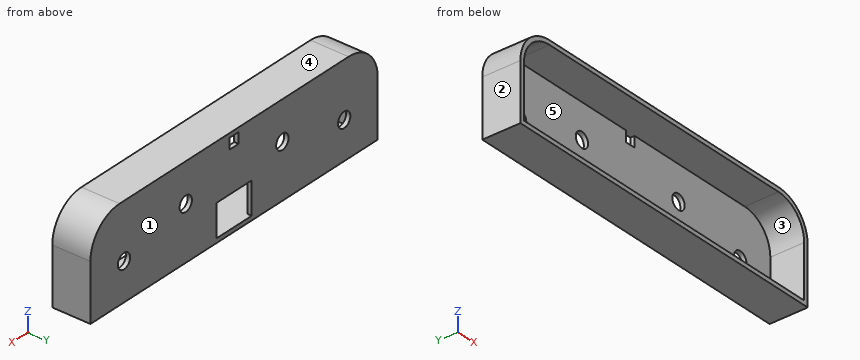
```python
from build123d import *

# Parameters (mm, degrees)
SKETCH1_W           = 162.7
SKETCH1_H           = 43
BOSS_EXTRUDE2_DEPTH = 17.75
FILLET2_R           = 16.5
SHELL1_T            = -2
SKETCH2_R           = 3.5
CUT_EXTRUDE1_DEPTH  = 86.994970783
SKETCH5_W           = 20
SKETCH5_H           = 15
CUT_EXTRUDE2_DEPTH  = 86.994970783
SKETCH6_W           = 5
SKETCH6_H           = 5
CUT_EXTRUDE3_DEPTH  = 86.994970783


with BuildPart() as part:
    # Sketch1 → Boss-Extrude2 (new body)
    with BuildSketch(Plane(origin=(0, 0, 0), x_dir=(1, 0, 0), z_dir=(0, 1, 0))):
        Rectangle(SKETCH1_W, SKETCH1_H)
    extrude(amount=BOSS_EXTRUDE2_DEPTH)

    # Fillet2
    fillet2_edges = [part.edges().sort_by_distance(p)[0] for p in [
        (81.35, 8.875, 21.5),
        (-81.35, 8.875, 21.5),
    ]]
    fillet(fillet2_edges, radius=FILLET2_R)

    # Shell1
    shell1_openings = [part.faces().sort_by_distance(p)[0] for p in [
        (0, 0, -0.302595299),
    ]]
    offset(amount=SHELL1_T, openings=shell1_openings, kind=Kind.INTERSECTION)

    # Sketch2 → Cut-Extrude1 (cut, through all)
    with BuildSketch(Plane(origin=(0, 17.75, 0), x_dir=(1, 0, 0), z_dir=(0, 1, 0))):
        with Locations(Location((-62.35, 4, 0), (0, 0, 270))):
            Circle(SKETCH2_R)
        with Locations(Location((-27.35, -3.5, 0), (0, 0, 270))):
            Circle(SKETCH2_R)
        with Locations(Location((27.35, -3.5, 0), (0, 0, 90))):
            Circle(SKETCH2_R)
        with Locations(Location((62.35, 4, 0), (0, 0, 90))):
            Circle(SKETCH2_R)
    extrude(amount=-CUT_EXTRUDE1_DEPTH, mode=Mode.SUBTRACT)

    # Sketch5 → Cut-Extrude2 (cut, through all)
    with BuildSketch(Plane(origin=(0, 17.75, 0), x_dir=(1, 0, 0), z_dir=(0, 1, 0))):
        with Locations((0, 12)):
            Rectangle(SKETCH5_W, SKETCH5_H)
    extrude(amount=-CUT_EXTRUDE2_DEPTH, mode=Mode.SUBTRACT)

    # Sketch6 → Cut-Extrude3 (cut, through all)
    with BuildSketch(Plane(origin=(0, 17.75, 0), x_dir=(1, 0, 0), z_dir=(0, 1, 0))):
        with Locations((0, -17)):
            Rectangle(SKETCH6_W, SKETCH6_H)
    extrude(amount=-CUT_EXTRUDE3_DEPTH, mode=Mode.SUBTRACT)


solid = part.part
```
Input: part model. Units: mm. Frame: model coordinates. Face numbers are marked on the shaded views. A direction names the side the tool comes from. Coordinates: 2 decimals unless noted, no trailing zeros. Write each loop counter-clockwise with the first axis right and the second up, starting at its lowest first coordinate (ties: lowest second). Pieces come first, ordered by that corner, then holes.
1) Section A-A on z = 3.5. Output: boundary loops of the cut face in (x, y).
2) Section B-B on x = -62.35. Output: boundary loops of the cut face in (y, z), and give its area (3 significant figures).
3) Section C-C on z = -12. Output: boundary loops of the cut face in (x, y), and give its area (3 significant figures).
4) Set-up query: the marked faces 4 and 5. Return all of +Z, -Z, +X, -X, +Y, -Y with unobstructed straight access to the full face (end or side cutting, diameter ignored); none if empty.
5) Section D-D on y = 3. Output: boundary loops of the cut face in (x, z).
6) Pin query (flat end, axial travel): pin 1 Ø1 at (y, z) = (16.5, 16.5) entering from -X; pin 2 Ø11.5 at (x, z) = (-39.5, 9.5) entering from -Y; pin 3 Ø4 at (x, z) = (-62.35, -4) entering from -Y. Return the tip coordinate at first contact, or that it passes through.
7) Mould query, pull axis X, two halves, no side actions, for the marked faces 1, 2 and 3. Classes: pulls with the +X half, pulls with the -X half, needs draft (parallel to the pull), parting line crosses it, or undercut.
8) Material intervals for line 1 along X through (y, z) = (16.8, -4); line 2 along X through (y, z) = (16.3, 3.5); line 3 along Z through (x, y) = (38, 13.75), sorted ascending.
Check result:
1. outline: (-81.35, 0) - (-79.35, 0) - (-79.35, 15.75) - (-30.85, 15.75) - (-30.85, 17.75) - (-81.35, 17.75) - close; (-23.85, 15.75) - (23.85, 15.75) - (23.85, 17.75) - (-23.85, 17.75) - close; (30.85, 15.75) - (79.35, 15.75) - (79.35, 0) - (81.35, 0) - (81.35, 17.75) - (30.85, 17.75) - close
2. outline: (0, -21.5) - (17.75, -21.5) - (17.75, -7.5) - (15.75, -7.5) - (15.75, -19.5) - (0, -19.5) - close; (0, 19.5) - (15.75, 19.5) - (15.75, -0.5) - (17.75, -0.5) - (17.75, 21.5) - (0, 21.5) - close
2. area: 135 mm2
3. outline: (-81.35, 0) - (-79.35, 0) - (-79.35, 15.75) - (-10, 15.75) - (-10, 17.75) - (-81.35, 17.75) - close; (10, 15.75) - (79.35, 15.75) - (79.35, 0) - (81.35, 0) - (81.35, 17.75) - (10, 17.75) - close
3. area: 348 mm2
4. face 4: +Z, +X, -X, +Y, -Y
4. face 5: -Y
5. outline: (-81.35, -21.5) - (81.35, -21.5) - (81.35, 5) arc R16.5 ccw to (64.85, 21.5) - (-64.85, 21.5) arc R16.5 ccw to (-81.35, 5) - close; hole (-79.35, -19.5) - (79.35, -19.5) - (79.35, 5) arc R14.5 ccw to (64.85, 19.5) - (-64.85, 19.5) arc R14.5 ccw to (-79.35, 5) - close
6. pin 1: stops at x = -77.15
6. pin 2: stops at y = 15.75
6. pin 3: passes through
7. face 1: needs draft
7. face 2: pulls with the -X half
7. face 3: undercut
8. line 1: x = -81.35 to -65.85, -58.85 to 58.85, 65.85 to 81.35
8. line 2: x = -81.35 to -30.85, -23.85 to 23.85, 30.85 to 81.35
8. line 3: z = -21.5 to -19.5, 19.5 to 21.5
